from build123d import *

# Parameters (mm, degrees)
BOSS_EXTRUDE1_DEPTH   = 6.25
BOSS_EXTRUDE2_DEPTH   = 5
BOSS_EXTRUDE3_START   = 28.7
BOSS_EXTRUDE3_DEPTH   = 28.7
SKETCH4_R             = 2.15
M4_THROUGH_HOLE_DEPTH = 47.541927843


with BuildPart() as part:
    # Sketch1 → Boss-Extrude1 (new body)
    with BuildSketch(Plane(origin=(0, 0, 0), x_dir=(1, 0, 0), z_dir=(0, 1, 0))):
        with BuildLine():
            ThreePointArc((33.093119943, -27.768424738), (18.257108907, -39.1524964), (0, -43.2))
            Line((0, -43.2), (0, -46.8))
            ThreePointArc((0, -46.8), (19.778534649, -42.415204433), (35.850879938, -30.082460133))
            Line((35.850879938, -30.082460133), (33.093119943, -27.768424738))
        make_face()
    extrude(amount=BOSS_EXTRUDE1_DEPTH)

    # Sketch2 → Boss-Extrude2 (add)
    with BuildSketch(Plane(origin=(0, 6.25, 0), x_dir=(1, 0, 0), z_dir=(0, 1, 0))):
        with BuildLine():
            ThreePointArc((35.850879938, -30.082460133), (19.778534649, -42.415204433), (0, -46.8))
            Line((0, -46.8), (0, -60))
            ThreePointArc((0, -60), (25.357095704, -54.378467222), (45.962666587, -38.567256581))
            Line((45.962666587, -38.567256581), (35.850879938, -30.082460133))
        make_face()
        with BuildLine():
            Line((35.850879938, -30.082460133), (33.093119943, -27.768424738))
            ThreePointArc((33.093119943, -27.768424738), (18.257108907, -39.1524964), (0, -43.2))
            Line((0, -43.2), (0, -46.8))
            ThreePointArc((0, -46.8), (19.778534649, -42.415204433), (35.850879938, -30.082460133))
        make_face()
        with BuildLine():
            ThreePointArc((30.794986613, -25.840061909), (16.989254122, -36.433573039), (0, -40.2))
            Line((0, -40.2), (0, -43.2))
            ThreePointArc((0, -43.2), (18.257108907, -39.1524964), (33.093119943, -27.768424738))
            Line((33.093119943, -27.768424738), (30.794986613, -25.840061909))
        make_face()
    extrude(amount=BOSS_EXTRUDE2_DEPTH)

    # Sketch3 → Boss-Extrude3 (add)
    with BuildSketch(Plane(origin=(0, 6.25, 0), x_dir=(-1, 0, 0), z_dir=(0, -1, 0)).offset(BOSS_EXTRUDE3_START)):
        with BuildLine():
            ThreePointArc((0, -55.2), (-23.328528048, -50.028189844), (-42.28565326, -35.481876055))
            Line((-42.28565326, -35.481876055), (-45.962666587, -38.567256581))
            ThreePointArc((-45.962666587, -38.567256581), (-25.357095704, -54.378467222), (0, -60))
            Line((0, -60), (0, -55.2))
        make_face()
    extrude(amount=-BOSS_EXTRUDE3_DEPTH)

    # Sketch4 → M4-through hole (cut, through all)
    with BuildSketch(Plane(origin=(15.397493307, 0, 33.020030955), x_dir=(0.9063077870366493, 0, -0.42261826174070105), z_dir=(0.42261826174070105, 0, 0.9063077870366493))):
        with Locations(Location((0, -14.95, 0), (0, 0, 180))):
            Circle(SKETCH4_R)
    extrude(amount=M4_THROUGH_HOLE_DEPTH, mode=Mode.SUBTRACT)


solid = part.part
Build history of the part. All positions in model axes, mm. A direction names the side the tool comes from. Coordinates: 2 decimals unless noted, no trailing zeros. Write each loop counter-clockwise with the first axis right and the second up, starting at its lowest first coordinate (ties: lowest second). Pieces come first, ordered by that corner, then holes.
(1) Drill centre lines: line 1 (Y direction, x = 9, z = 47); line 2 (Z direction, x = 17.5, y = -20); line 3 (Z direction, x = 11, y = -10.5). Where is each one in solid material? Low to high.
(2) Cut at C-C on z = 46. List the corners of the cut face in (x, y), and give its area (3 significant figures).
(3) Cut at A-A on y = 1. List the corners of the cut face in (x, z).
(4) Mould opens along Y. For faces 1 (the flat face through (18, 11.25, 46)), 2 (the flat face through (23.1, -22.45, 50.4)), 3 (the cylindrical face through (25.866, -13.642, 51.432)) say: pulls with the +Y half, pulls with the -Y half, needs draft (parallel to the pull), parting line crosses it, or undercut.
(5) 3-axis set-ups, long thin cutter, end or side, ignore diameter. For faces 4 (the cylindrical face through (25.69, -5.84, 54.22)), 5 (the cylindrical face through (18.5, 3.08, 39.04)), 6 (the flat face through (21, 6.25, 45)): which of +Z, -Z, +X, -X, +Y, -Y reach the whole face in a straight line?
(6) Cut at D-D on y = -13.5. List the corners of the cut face in (x, z), and give its area (3 significant figures).
(7) Pin check, flat tips, straight feed: pin 1 Ø5 at (x, z) = (41, 32) entering from -Y; pin 2 Ø14 at (x, z) = (22.5, 32) entering from -Y; pin 3 Ø12 at (x, y) = (39.5, -18.5) entering from -Z. Stop position of each tip, or through.
(8) Cut at B-B on x = 30. List the corners of the cut face in (y, z).
Working result:
1. line 1: y = 6.25 to 11.25
1. line 2: z = 52.35 to 57.39
1. line 3: z = 54.09 to 58.98
2. outline: (0, 0) - (8.62, 0) - (8.62, 6.25) - (30.51, 6.25) - (30.51, -22.45) - (38.52, -22.45) - (38.52, 11.25) - (0, 11.25) - close
2. area: 476 mm2
3. outline: (0, 43.2) arc R43.2 cw to (33.09, 27.77) - (35.85, 30.08) arc R46.8 ccw to (0, 46.8) - close; (0, 55.2) arc R55.2 cw to (42.29, 35.48) - (45.96, 38.57) arc R60 ccw to (0, 60) - close
4. face 1: pulls with the +Y half
4. face 2: pulls with the -Y half
4. face 3: undercut
5. face 4: +Z, +X, +Y, -Y
5. face 5: -Z, -X, -Y
5. face 6: -Y
6. outline: (0, 55.2) arc R55.2 cw to (21.88, 50.68) - (23.91, 55.03) arc R60 ccw to (0, 60) - close; (24.76, 49.34) arc R55.2 cw to (42.29, 35.48) - (45.96, 38.57) arc R60 ccw to (26.79, 53.69) - close
6. area: 226 mm2
7. pin 1: stops at y = 6.25
7. pin 2: stops at y = 0
7. pin 3: stops at z = 35.48
8. outline: (-22.45, 46.34) - (6.25, 46.34) - (6.25, 35.92) - (0, 35.92) - (0, 31.08) - (6.25, 31.08) - (6.25, 26.76) - (11.25, 26.76) - (11.25, 51.96) - (-22.45, 51.96) - close
